Verification items for this drawing (mm, ordinates from the low corner). Round coordinates to 2 decimals unless told otherwise and drop trailing zeros. Loops run counter-clockwise (first coordinate to the right, second up) from the corner with the lowest first, then second, coordinate; pieces in that order, holes last. Notation, with made-up numbers: (13, 75.5) -> (60, 75.5) arc R26 ccw to (60, 104.5) -> close; hole circle Ø9 at (53, 56.5). An arc over 180 degrees is marked (long way). One line per item, written item: value. Start each with the question number.
1. Go/stop test with flat-tipped pins: pin 1 (1 mm diameter, centred on x = 14, z = 27, fed in from -Y); pin 2 (6 mm diameter, centred on x = 4.5, z = 14, fed in from +Y); pin 3 (6 mm diameter, centred on y = 17.5, z = 78, fed in from -X). Record where each tip stops, or that it passes through.
2. Material ranges on L1, parallel to Z at x = 15.75, y = 18.25; L2, parallel to Z at x = 11.5, y = 18; L3, parallel to X at y = 17.75, z = 23, recorded low to high.
3. Release check for a two-part mould opening along X. For the marked faces 1 and 2 record: +X half, -X half, draft (parallel to the pull), parting line (faces both ways), or undercut.
4. Cross-section at C-C on z = 9.5. Record the cut outline in (x, y).
5. Cross-section at A-A on x = 10.5. Record the cut outline in (y, z).
6. Cross-section at D-D on z = 54. Record the cut outline in (x, y).
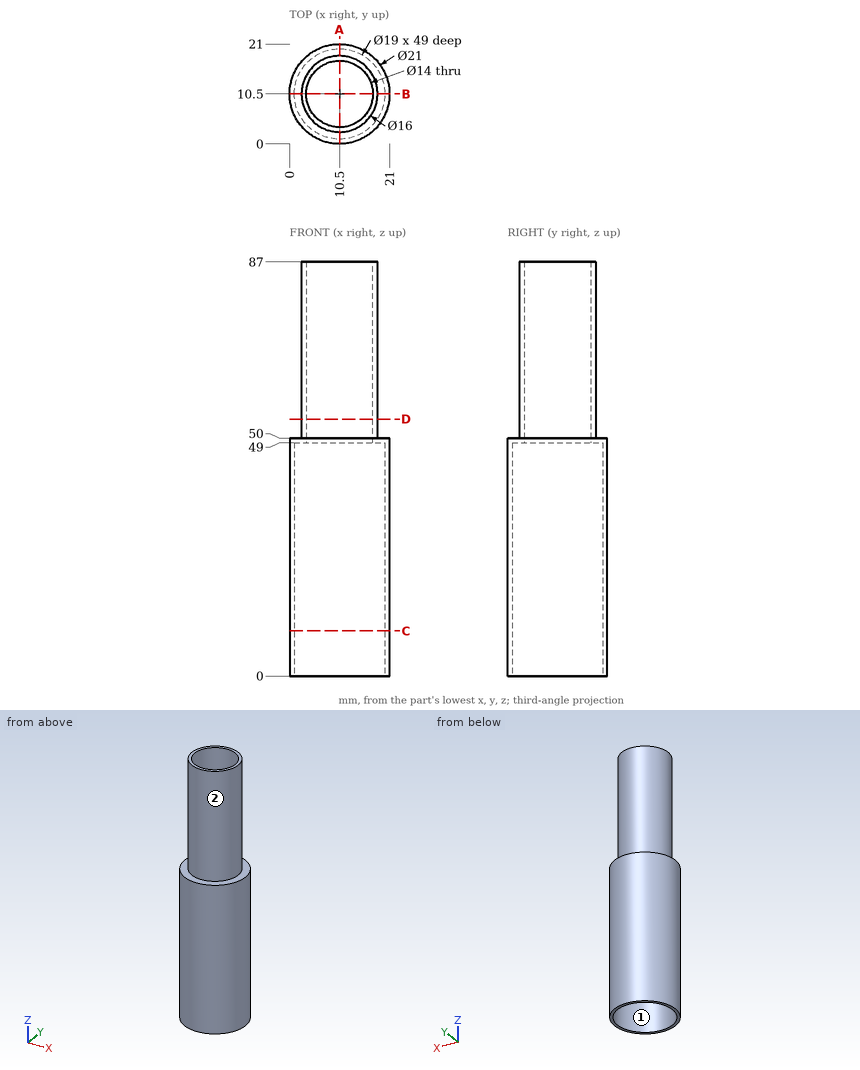
Taken from the geometry:
1. pin 1: stops at y = 0.44
1. pin 2: stops at y = 20.56
1. pin 3: stops at x = 3.57
2. L1: z = 49 to 50
2. L2: z = 49 to 87
2. L3: x = 2.9 to 4.36, 16.64 to 18.1
3. face 1: undercut
3. face 2: parting line
4. outline: circle Ø21 at (10.5, 10.5); hole circle Ø19 at (10.5, 10.5)
5. outline: (0, 0) -> (1, 0) -> (1, 49) -> (3.5, 49) -> (3.5, 87) -> (2.5, 87) -> (2.5, 50) -> (0, 50) -> close; (17.5, 49) -> (20, 49) -> (20, 0) -> (21, 0) -> (21, 50) -> (18.5, 50) -> (18.5, 87) -> (17.5, 87) -> close
6. outline: circle Ø16 at (10.5, 10.5); hole circle Ø14 at (10.5, 10.5)
